Build history of the part. All positions in model axes, mm. A direction names the side the tool comes from. Round coordinates to 2 decimals unless told otherwise and drop trailing zeros. Loops run counter-clockwise (first coordinate to the right, second up) from the corner with the lowest first, then second, coordinate; pieces in that order, holes last. Notation, with made-up numbers: (-8, 20) - (30, 20) arc R13 cw to (30, 26) - close; hole circle Ø11 at (14, -22). An arc over 180 degrees is marked (long way). One line per question, with ' | ' between items. Start each with the question number.
from build123d import *


with BuildPart() as f1:
    # F0 (on Front) → F1 (revolve)
    with BuildSketch(Plane.XZ):
        Polygon((-29.822183, -23.230489), (-55.222183, -23.230489), (-55.222183, -35.930488), (-21.117112, -35.930488), (-19.040657, -30.561369), (-15.62502, -21.72951), (-12.072363, -12.543354), (-9.076869, -4.797863), (-5.045252, 5.626746), (-2.506006, 12.19251), (2.118304, 24.149653), (-11.49837, 24.149653), align=None)
        Polygon((2.118304, 17.961016), (2.118304, 24.149653), (-2.506006, 12.19251), (0, 12.19251), (0, 17.961016), align=None)
        Polygon((-15.62502, -21.72951), (-19.040657, -30.561369), (-15.62502, -30.561369), align=None)
        Polygon((-2.506006, 4.644717), (-2.506006, 12.19251), (-5.045252, 5.626746), align=None)
        Polygon((-12.072363, -12.543354), (-15.62502, -21.72951), (-12.072363, -21.72951), align=None)
        Polygon((-5.045252, -4.797863), (-5.045252, 5.626746), (-9.076869, -4.797863), align=None)
        Polygon((-9.076869, -4.797863), (-12.072363, -12.543354), (-9.076869, -12.543354), align=None)
    revolve(axis=Axis((-55.222183, 0, -5.890418), (0, 0, 1)))


solid = f1.part
1) Drop flat-ended pins along their axis: pin 1 (1.5 mm diameter, centred on y = -5, z = 1.5, fed in from -X); pin 2 (4 mm diameter, centred on x = -25, z = -6, fed in from +Y); pin 3 (5 mm diameter, centred on x = -36, z = -2.5, fed in from +Y). Give the stop position or say it passes through.
2) Wall check: line 1 (Y direction, x = -64, z = -19); line 2 (Y direction, x = -29, z = 20); line 3 (X direction, y = -23, z = 14). Give the ranges that are in metal, low to high. Write a range as [from, to].
3) Tool access for faces 5 (the cylindrical face through (-98.33, 1.9, -17.07)), 6 (the conical face through (-26.26, 9.12, -10.4)): list every direction of +Z, -Z, +X, -X, +Y, -Y with a clear straight run to the whole face (end or side of a thin tool).
4) Saw through at A-A on z = -15. Write the cut outline in (x, y), and give its area (3 significant figures).
5) Two-plate mould, pull along Y, no slides. Class faces 1 (the cylindrical face through (-4.94, 15.83, 8.47)), 2 (the flat face through (-25, 47, 17.961)), 3 (the conical face through (-92.322, 34.019, 5.565)), 4 (the flat face through (-56, 0, -23.23)): +Y half, -Y half, draft (parallel to the pull), parting line (faces both ways), or undercut.
Answer key:
1) pin 1: x = -105.22 | pin 2: y = 41.21 | pin 3: y = 47.31
2) line 1: [-42.25, -25.57], [25.57, 42.25] | line 2: [-50.99, -32.96], [32.96, 50.99] | line 3: [-105.43, -87.7], [-22.74, -5.02]
3) face 5: -Z | face 6: +Z
4) outline: circle Ø86.3 at (-55.22, 0); hole circle Ø57.17 at (-55.22, 0) | area: 3,280 mm²
5) face 1: parting line | face 2: draft | face 3: undercut | face 4: undercut
